Autodesk Inventor part; units mm, degrees
ref_plane "YZ Plane" through (0, 0, 0) normal (1, 0, 0) x (0, 1, 0)
ref_plane "XZ Plane" through (0, 0, 0) normal (0, 1, 0) x (-1, 0, 0)
ref_plane "XY Plane" through (0, 0, 0) normal (0, 0, 1) x (1, 0, 0)
sketch "Sketch1" plane through (0, 0, 0) normal (0, 1, 0) x (-1, 0, 0)
  circle A0 centre (0, 0) radius 10
  line L0 (0, 28) -> (0, -28) construction
  line L1 (-5.5, 28) -> (-5.5, -28)
  line L2 (5.5, -28) -> (5.5, 28)
  arc A1 (5.5, 28) -> (-5.5, 28) centre (0, 28) ccw
  arc A2 (-5.5, -28) -> (5.5, -28) centre (0, -28) ccw
  circle A3 centre (0, 0) radius 5
  circle A4 centre (0, 28) radius 2.75
  circle A5 centre (0, -28) radius 2.75
  point P0 (-5.5, 8.3516)
  point P1 (-5.5, -8.3516)
  point P2 (5.5, -8.3516)
  point P3 (5.5, 8.3516)
  dimension "d0" = 56
  dimension "d1" = 20
  dimension "d2" = 10
  dimension "d3" = 5.5
  dimension "d4" = 5.5
extrude "Extrusion1" add sketch "Sketch1" along normal blind 1.5
ref_plane "Work Plane1" through (0, 6.5, 0) normal (0, 1, 0) x (1, 0, 0)
sketch "Sketch4" plane through (0, 1.5, 0) normal (0, 1, 0) x (1, 0, 0)
  arc A0 (5.5, -8.3516) -> (5.5, 8.3516) centre (0, 0) ccw
  circle A1 centre (0, 0) radius 10
sketch "Sketch2" plane through (0, 6.5, 0) normal (0, 1, 0) x (1, 0, 0)
  circle A0 centre (0, 0) radius 5
  circle A1 centre (0, 0) radius 5
loft "Loft2" add profiles "Sketch2", "Sketch4"
sketch "Sketch3" plane through (0, 0, 0) normal (0, -1, 0) x (1, 0, 0)
  circle A0 centre (0, 0) radius 5
  circle A1 centre (0, 28) radius 2.75
  circle A2 centre (0, -28) radius 2.75
extrude "Extrusion2" cut sketch "Sketch3" against normal through all
mirror "Mirror1" about plane through (0, 0, 0) normal (0, -1, 0) of "Extrusion1", "Loft2", "Extrusion2"
properties part number "12_Thong_lo_xo"
Part model, mm, in its own coordinate system. A direction names the side the tool comes from. Round coordinates to 2 decimals unless told otherwise and drop trailing zeros. Write each loop counter-clockwise with the first axis right and the second up, starting at its lowest first coordinate (ties: lowest second). Pieces come first, ordered by that corner, then holes.
Item 1: Cut at B-B, the plane z = -15. Give the cut face in (x, y).
Results:
outline: (-5.5, -1.5) - (5.5, -1.5) - (5.5, 1.5) - (-5.5, 1.5) - close
Item 2: Which spindle directions (+Z, -Z, +X, -X, +Y, -Y) get a long thin tool onto all of the face, cutting with end or side? Do faces 4 (the flat face through (5.5, 0, -18)), 5 (the flat face through (5.5, 0, 18)), 6 (the flat face through (-5.5, 0, -18)). Say none if no direction does.
Results:
face 4: -Z, +X, +Y, -Y
face 5: +Z, +X, +Y, -Y
face 6: -Z, -X, +Y, -Y
Item 3: Probe L1, parallel to Z at x = 0, y = 0.85; L2, parallel to X at y = 0.3, z = -28; L3, parallel to Z at x = 0, y = 3.3. List the from-to ranges inside material, lowest first.
Results:
L1: z = -33.5 to -30.75, -25.25 to -5, 5 to 25.25, 30.75 to 33.5
L2: x = -5.5 to -2.75, 2.75 to 5.5
L3: z = -8.2 to -5, 5 to 8.2
Item 4: Two-plate mould, pull along X, no slides. Class faces 1 (the cylindrical face through (0.358, 0.021, 30.727)), 2 (the cylindrical face through (-0.1, 0, 33.5)), 3 (the flat face through (0, -1.5, 21)): +X half, -X half, draft (parallel to the pull), parting line (faces both ways), or undercut.
Results:
face 1: undercut
face 2: parting line
face 3: draft
Item 5: Cut at A-A, the plane x = 0. Count the separate pieces of the cut face and the enclosed holes in it, plus the area to 3 significant figures.
Results:
separate pieces: 4
enclosed holes: 0
area: 188 mm2
Item 6: Drop flat-ended pins along their axis: pin 1 Ø6 at (x, y) = (-4.5, 1.5) entering from +Z; pin 2 Ø12 at (x, z) = (0, 27) entering from -Y; pin 3 Ø11.5 at (x, z) = (0, 0) entering from +Y; pin 4 Ø9 at (x, z) = (-1, -24) entering from +Y. Give the stop position or say it passes through.
Results:
pin 1: stops at z = 33.29
pin 2: stops at y = -1.5
pin 3: stops at y = 6.5
pin 4: stops at y = 1.5
